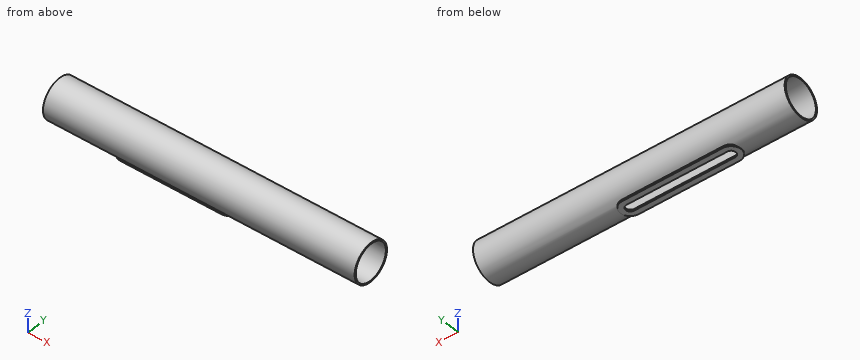
```python
from build123d import *

# Parameters (mm, degrees)
SKETCH005_R     = 10.75
SKETCH005_R_2   = 10
PAD001_DEPTH    = 170
POCKET013_DEPTH = 5
PAD009_DEPTH    = 1


with BuildPart() as part:
    # Sketch005 → Pad001 (new body)
    with BuildSketch(Plane.YZ):
        Circle(SKETCH005_R)
        Circle(SKETCH005_R_2, mode=Mode.SUBTRACT)
    extrude(amount=PAD001_DEPTH)

    # Sketch021 (on DatumPlane) → Pocket013 (cut)
    with BuildSketch(Plane.YX.offset(11)):
        with BuildLine():
            ThreePointArc((3.5, 93), (0, 96.5), (-3.5, 93))
            Line((-3.5, 93), (-3.5, 38))
            ThreePointArc((-3.5, 38), (0, 34.5), (3.5, 38))
            Line((3.5, 38), (3.5, 93))
        make_face()
    extrude(amount=-POCKET013_DEPTH, mode=Mode.SUBTRACT)

    # Sketch026 (on DatumPlane) → Pad009 (join)
    with BuildSketch(Plane.YX.offset(11)):
        with BuildLine():
            ThreePointArc((5.5, 93), (0, 98.5), (-5.5, 93))
            Line((-5.5, 93), (-5.5, 38))
            ThreePointArc((-5.5, 38), (0, 32.5), (5.5, 38))
            Line((5.5, 38), (5.5, 93))
        make_face()
        with BuildLine():
            ThreePointArc((-2.5, 38), (0, 35.5), (2.5, 38))
            Line((2.5, 38), (2.5, 93))
            ThreePointArc((2.5, 93), (0, 95.5), (-2.5, 93))
            Line((-2.5, 93), (-2.5, 38))
        make_face(mode=Mode.SUBTRACT)
    extrude(amount=-PAD009_DEPTH)


solid = part.part
```
Check sheet for the modelled part. Datum: model origin and axes. Units: mm. Give positions to 0.01 mm unless a question says otherwise; leave off trailing zeros. Write each loop counter-clockwise with the first axis right and the second up, starting at its lowest first coordinate (ties: lowest second). Pieces come first, ordered by that corner, then holes. Notation, with made-up numbers: (-35.5, -37.5) - (-23.5, -37.5) arc R35 ccw to (-23.5, -5.5) - close; hole circle Ø10 at (38, 54.5). An arc over 180 degrees is marked (long way). Answer as a JSON object with one key per item and string values. Group by question number.
1) Sectioned sample at D-D (x = 103.5). Record the cut outline in (y, z).
2) Depth check by flat-ended pin: P1, Ø4, axis at x = 54, z = -1, coming from the -Y side; P2, Ø1.5, axis at x = 124.5, y = -3.5, coming from the -Z side; P3, Ø6, axis at x = 53.5, y = -6.5, coming from the +Z side; P4, Ø4, axis at x = 27.5, y = -6.5, coming from the +Z side. Enter the tip coordinate at first touch or a pass-through.
3) Thickness scan on probe 1 along Z at (x, y) = (126, 0); probe 2 along Z at (x, y) = (41.5, 0); probe 3 along Z at (x, y) = (81.5, 3). Record the ranges inside material, lowest first. Write a range as from..to.
4) Sectioned sample at C-C (z = 8.25). Record the cut outline in (x, y).
5) Sectioned sample at A-A (z = 0). Record the cut outline in (x, y), then the cut area to 3 significant figures.
6) Sectioned sample at B-B (x = 74). Record the cut outline in (y, z), then the cut area to 3 significant figures.
Geometry results:
{
 "1": {"outline": "circle Ø21.5 at (0, 0); hole circle Ø20 at (0, 0)"},
 "2": {"P1": "stops at y = -10.75", "P2": "stops at z = -10.39", "P3": "stops at z = 10.16", "P4": "stops at z = 9.76"},
 "3": {"probe 1": "z = -10.75..-10, 10..10.75", "probe 2": "z = 10..10.75", "probe 3": "z = -11..-10, 9.54..10.32"},
 "4": {"outline": "(0, -6.89) - (170, -6.89) - (170, -5.65) - (0, -5.65) - close; (0, 5.65) - (170, 5.65) - (170, 6.89) - (0, 6.89) - close"},
 "5": {"outline": "(0, -10.75) - (170, -10.75) - (170, -10) - (0, -10) - close; (0, 10) - (170, 10) - (170, 10.75) - (0, 10.75) - close", "area": "255 mm^2"},
 "6": {"outline": "(-5.5, -11) - (-2.5, -11) - (-2.5, -10) - (-3.5, -10) - (-3.5, -9.37) arc R10 cw (long way) to (3.5, -9.37) - (3.5, -10) - (2.5, -10) - (2.5, -11) - (5.5, -11) - (5.5, -10) - (3.94, -10) arc R10.75 ccw (long way) to (-3.94, -10) - (-5.5, -10) - close", "area": "49.5 mm^2"}
}
